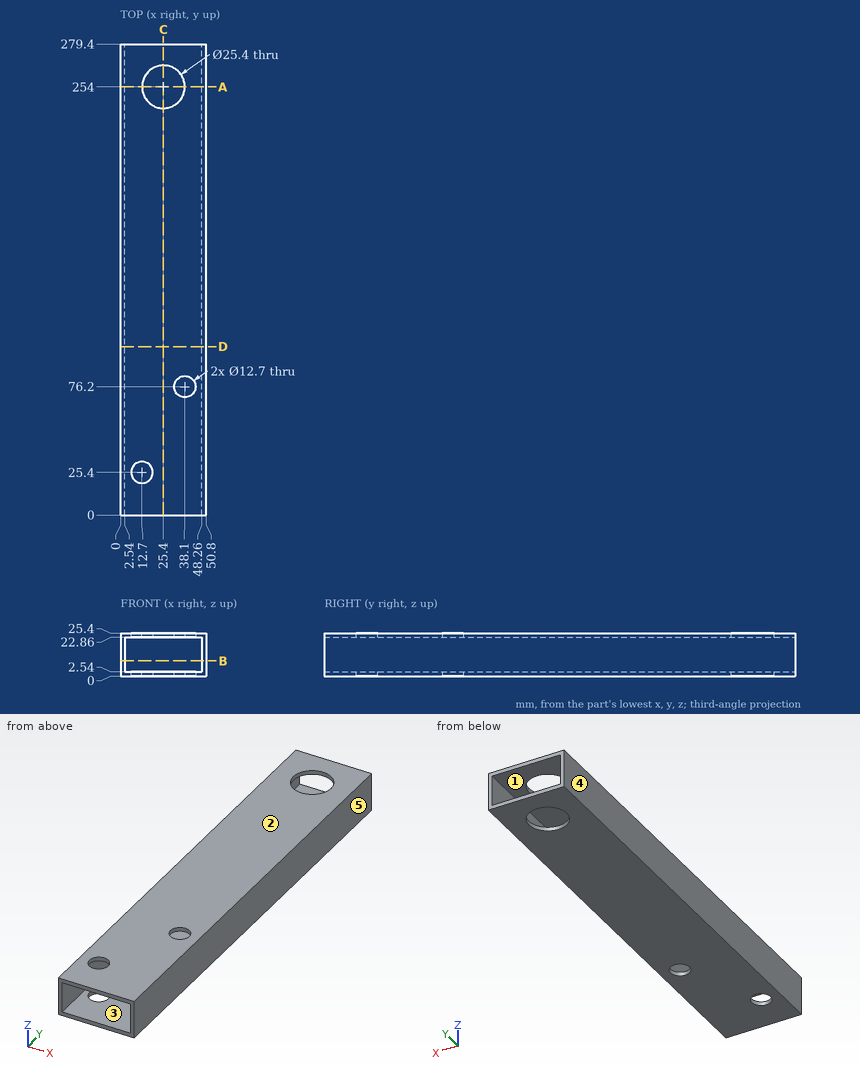
Print and shaded views of the part. All mm, measured from the part's lowest x, y and z. A direction names the side the tool comes from. Coordinates: 2 decimals unless noted, no trailing zeros. Order: outer loops, then holes, each group sorted by start corner. A loop starts at its lowest first (then second) coordinate and runs counter-clockwise, first axis right, second up. Notation, with made-up numbers: (-11.75, 89.25) -> (17.25, 89.25) arc R36 ccw to (17.25, 124.25) -> close; hole circle Ø8 at (79.5, 74). An arc over 180 degrees is marked (long way). Answer as a JSON object with one key per item and string values. Group by question number.
1) Cut at B-B, the plane z = 9. Write the cut outline in (x, y).
2) Which spindle directions (+Z, -Z, +X, -X, +Y, -Y) get a long thin tool onto all of the face, cutting with end or side? Do the marked faces 1 and 2. Say none if no direction does.
3) Flat gauge pin, fed straight in: pin 1 (7.5 mm diameter, centred on x = 12.7, y = 25.4, fed in from -Z). Where does the tip first touch, or does it go through?
4) Pull direction X, two halves, no side cores. Call the marked faces 3, 4 and 5: +X half, -X half, draft (parallel to the pull), parting line (faces both ways), or undercut.
5) Cut at A-A, the plane y = 254. Write the cut outline in (x, z).
6) Cut at D-D, the plane y = 100. Write the cut outline in (x, z).
7) Cut at C-C, the plane x = 25.4. Write the cut outline in (y, z), then the cut area to 3 significant figures.
8) Drill centre lines: L1, parallel to X at y = 246, z = 3.5; L2, parallel to Z at x = 21, y = 124.5; L3, parallel to Y at x = 25.4, z = 24. Where is each one in solid material? Low to high.
Check values:
{
 "1": {"outline": "(0, 0) -> (2.54, 0) -> (2.54, 279.4) -> (0, 279.4) -> close; (48.26, 0) -> (50.8, 0) -> (50.8, 279.4) -> (48.26, 279.4) -> close"},
 "2": {"face 1": "+Y, -Y", "face 2": "+Z, +X, -X, +Y, -Y"},
 "3": {"pin 1": "passes through"},
 "4": {"face 3": "undercut", "face 4": "-X half", "face 5": "+X half"},
 "5": {"outline": "(0, 0) -> (12.7, 0) -> (12.7, 2.54) -> (2.54, 2.54) -> (2.54, 22.86) -> (12.7, 22.86) -> (12.7, 25.4) -> (0, 25.4) -> close; (38.1, 0) -> (50.8, 0) -> (50.8, 25.4) -> (38.1, 25.4) -> (38.1, 22.86) -> (48.26, 22.86) -> (48.26, 2.54) -> (38.1, 2.54) -> close"},
 "6": {"outline": "(0, 0) -> (50.8, 0) -> (50.8, 25.4) -> (0, 25.4) -> close; hole (2.54, 2.54) -> (48.26, 2.54) -> (48.26, 22.86) -> (2.54, 22.86) -> close"},
 "7": {"outline": "(0, 0) -> (241.3, 0) -> (241.3, 2.54) -> (0, 2.54) -> close; (0, 22.86) -> (241.3, 22.86) -> (241.3, 25.4) -> (0, 25.4) -> close; (266.7, 0) -> (279.4, 0) -> (279.4, 2.54) -> (266.7, 2.54) -> close; (266.7, 22.86) -> (279.4, 22.86) -> (279.4, 25.4) -> (266.7, 25.4) -> close", "area": "1,290 mm²"},
 "8": {"L1": "x = 0 to 2.54, 48.26 to 50.8", "L2": "z = 0 to 2.54, 22.86 to 25.4", "L3": "y = 0 to 241.3, 266.7 to 279.4"}
}
